from build123d import *

# Parameters (mm, degrees)
F1_DEPTH = 63.5
F0_W     = 25.4
F0_H     = 19.05
F2_DEPTH = 25.4
F3_DEPTH = 8.5725
F5_R     = 6.35


with BuildPart() as f1:
    # F0 (on Front) → F1 (new body, symmetric)
    with BuildSketch(Plane.XZ):
        Polygon((-41.275, 9.525), (-41.275, -9.525), (41.275, -9.525), (41.275, 9.525), (22.225, 9.525), align=None)
    extrude(amount=F1_DEPTH, both=True)

    # F0 (on Front) → F2 (join, symmetric)
    with BuildSketch(Plane.XZ):
        with BuildLine():
            Line((22.225, 9.525), (41.275, 9.525))
            Line((41.275, 9.525), (41.275, 27.0002))
            ThreePointArc((41.275, 27.0002), (45.9246798487, 38.2255201513), (57.15, 42.8752))
            Line((57.15, 42.8752), (60.325, 42.8752))
            Line((60.325, 42.8752), (60.325, 61.9252))
            Line((60.325, 61.9252), (57.15, 61.9252))
            add(Edge.make_bspline(
                [(56.1238979845, 61.9101232261), (56.4661986033, 61.9166358314), (56.8082401142, 61.9216656861), (57.15, 61.9252)],
                knots=[110.6863449834, 110.6863449834, 110.6863449834, 110.6863449834, 111.5045361635, 111.5045361635, 111.5045361635, 111.5045361635], degree=3))
            ThreePointArc((56.1238979845, 61.9101232261), (32.0941400278, 51.3304179615), (22.225, 27.0002))
            Line((22.225, 27.0002), (22.225, 9.525))
        make_face()
        with Locations((73.025, 52.4002)):
            Rectangle(F0_W, F0_H)
    extrude(amount=F2_DEPTH, both=True)

    # F0 (on Front) → F3 (join, symmetric)
    with BuildSketch(Plane.XZ):
        with BuildLine():
            add(Edge.make_bspline(
                [(-41.275, 9.525), (-41.2321390497, 33.0120007106), (9.8168669335, 61.0290865026), (56.1238979845, 61.9101232261)],
                knots=[0, 0, 0, 0, 110.6863449834, 110.6863449834, 110.6863449834, 110.6863449834], degree=3))
            Line((-41.275, 9.525), (22.225, 9.525))
            Line((22.225, 9.525), (22.225, 27.0002))
            ThreePointArc((22.225, 27.0002), (32.0941400278, 51.3304179615), (56.1238979845, 61.9101232261))
        make_face()
    extrude(amount=F3_DEPTH, both=True)

    # F0 (on Front) → F4 (revolve)
    with BuildSketch(Plane.XZ):
        Polygon((85.725, 66.675), (85.725, 61.9252), (85.725, 42.8752), (85.725, 38.1), (111.125, 38.1), (111.125, 66.675), align=None)
    revolve(axis=Axis((85.725, 0, 52.3875), (0, 0, 1)))

    # F5
    f5_edges = [f1.edges().sort_by_distance(p)[0] for p in [
        (-41.275, -63.5, 0),
        (41.275, -63.5, 0),
        (41.275, 63.5, 0),
        (-41.275, 63.5, 0),
    ]]
    fillet(f5_edges, radius=F5_R)


solid = f1.part
Geometry: final body of the model. Coordinates: model frame, mm. A direction names the side the tool comes from. Give positions to 0.01 mm unless a question says otherwise; leave off trailing zeros. Loops run counter-clockwise (first coordinate to the right, second up) from the corner with the lowest first, then second, coordinate; pieces in that order, holes last. Notation, with made-up numbers: (54, 86.25) - (58, 86.25) arc R11 cw to (58, 97.25) - close; hole circle Ø4 at (68.5, 86.25). An arc over 180 degrees is marked (long way). One line per question, with ' | ' between items. Start each with the question number.
(1) Contact query for flat-ended pins moving along their axis: pin 1 (1.5 mm diameter, centred on x = 42, z = 41, fed in from -Y); pin 2 (11 mm diameter, centred on y = 25, z = 13.5, fed in from +X) (3 decimals); pin 3 (8 mm diameter, centred on y = 6, z = 33, fed in from +X). Output: stop coordinate, or through.
(2) Section query B-B on y = 42. Return loops of the section in (x, z) (3 decimals).
(3) Reachability of faces 1 (the flat face through (41.275, -1, 4)), 2 (the flat face through (22.225, 17, 18)), 3 (the flat face through (60, -2, 61.925)) from +Z, -Z, +X, -X, +Y, -Y: full face, straight path, thin tool, end or side. Return the list, or none.
(4) Ray query, line 1 (Y direction, x = 47.5, z = 57); line 2 (Y direction, x = -19, z = 27); line 3 (Z direction, x = -27.5, y = 20) (3 decimals). Return the intervals inside material, ascending. Write a range as from..to.
(5) Section query A-A on z = -3. Return loops of the section in (x, y) (3 decimals), then the cut area to 3 significant figures.
(6) Pull-direction query (X, two-part tool) for faces 4 (the flat face through (0, -63.5, 0)), 5 (the flat face through (22.225, -17, 18)), 6 (the flat face through (60, 2, 42.875)); classes: released by +X, released by -X, zero draft, split by the parting line, or undercut.
The answers:
1) pin 1: y = -25.4 | pin 2: x = 41.275 | pin 3: x = 44.82
2) outline: (-41.275, -9.525) - (41.275, -9.525) - (41.275, 9.525) - (-41.275, 9.525) - close
3) face 1: -Z, +X, +Y, -Y | face 2: +Z, -X, +Y | face 3: +Z, -X
4) line 1: -25.4..25.4 | line 2: -8.57..8.57 | line 3: -9.525..9.525
5) outline: (-41.275, -57.15) arc R6.35 ccw to (-34.925, -63.5) - (34.925, -63.5) arc R6.35 ccw to (41.275, -57.15) - (41.275, 57.15) arc R6.35 ccw to (34.925, 63.5) - (-34.925, 63.5) arc R6.35 ccw to (-41.275, 57.15) - close | area: 10,400 mm2
6) face 4: zero draft | face 5: released by -X | face 6: undercut
